```python
from build123d import *

# Parameters (mm, degrees)
SKETCH1_W           = 200
SKETCH1_H           = 30
BOSS_EXTRUDE1_DEPTH = 10
SKETCH2_R           = 5.125
CUT_EXTRUDE1_DEPTH  = 102.612007165


with BuildPart() as part:
    # Sketch1 → Boss-Extrude1 (new body)
    with BuildSketch(Plane(origin=(0, 0, 0), x_dir=(1, 0, 0), z_dir=(0, 1, 0))):
        Rectangle(SKETCH1_W, SKETCH1_H)
    extrude(amount=BOSS_EXTRUDE1_DEPTH)

    # Sketch2 → Cut-Extrude1 (cut, through all)
    with BuildSketch(Plane(origin=(0, 10, 0), x_dir=(1, 0, 0), z_dir=(0, 1, 0))):
        with Locations(Location((84, 0, 0), (0, 0, 270))):
            Circle(SKETCH2_R)
    extrude(amount=-CUT_EXTRUDE1_DEPTH, mode=Mode.SUBTRACT)


solid = part.part
```
Here's how the part is built. I have some questions about the finished solid (model axes, mm). Round coordinates to 2 decimals unless told otherwise and drop trailing zeros. Order: outer loops, then holes, each group sorted by start corner. A loop starts at its lowest first (then second) coordinate and runs counter-clockwise, first axis right, second up. Notation, with made-up numbers: M 66,10.5 L 106,10.5 A18 cw 106,33.5 Z; hole C -35,12.25 d3. An arc over 180 degrees is marked long. Answer in a Markdown table with one row per item.
Item 1: Imagine slicing it at B-B, the plane x = 84. Write out the boundary of the cut face in (y, z) (3 decimals), and give its area (4 significant figures).
A:
| item | result |
|---|---|
| outline | M 0,-15 L 10,-15 L 10,-5.125 L 0,-5.125 Z; M 0,5.125 L 10,5.125 L 10,15 L 0,15 Z |
| area | 197.5 mm2 |
Item 2: Thinking about a two-plate mould opening in X: for faces 1 (the face through (78.997, 5.07, -1.111)), 2 (the face through (100, 5, 0)), 3 (the face through (-1, 10, 0)), which applies, +X half, -X half, draft (parallel to the pull), parting line (faces both ways), or undercut?
A:
| item | result |
|---|---|
| face 1 | undercut |
| face 2 | +X half |
| face 3 | draft |
Item 3: If I drill on L1, parallel to X at y = 3, z = 0 (3 decimals); L2, parallel to X at y = 2.25, z = 3, over which ranges is the centre line in solid material (lowest first)? Write a range as from..to.
A:
| item | result |
|---|---|
| L1 | x = -100..78.875, 89.125..100 |
| L2 | x = -100..79.84, 88.16..100 |
Item 4: Imagine slicing it at A-A, the plane z = 0. Write out the boundary of the cut face in (x, y) (3 decimals), and give its area (3 significant figures).
A:
| item | result |
|---|---|
| outline | M -100,0 L 78.875,0 L 78.875,10 L -100,10 Z; M 89.125,0 L 100,0 L 100,10 L 89.125,10 Z |
| area | 1,900 mm2 |
